Check sheet for the modelled part. Datum: model origin and axes. Units: mm. Give positions to 0.01 mm unless a question says otherwise; leave off trailing zeros. Loops run counter-clockwise (first coordinate to the right, second up) from the corner with the lowest first, then second, coordinate; pieces in that order, holes last. Notation, with made-up numbers: (40.25, 49.25) - (48.25, 49.25) arc R27 cw to (48.25, 85.25) - close; hole circle Ø1 at (43, -3.5). An arc over 180 degrees is marked (long way). Answer in a Markdown table with one row per item. Add a question column.
(1) Sectioned sample at B-B on x = -10.5. Enter the section's corners in (y, z).
(2) Thickness scan on L1, parallel to Y at x = 2, z = -46.5; L2, parallel to X at y = 28, z = -70.5; L3, parallel to Z at x = 0, y = 30. Record the ranges inside material, lowest first.
(3) Sectioned sample at D-D on x = 3. Enter the section's corners in (y, z).
(4) Go/stop test with flat-tipped pins: P1, Ø1.7, axis at x = 22.5, z = 32, coming from the +Y side; P2, Ø2, axis at x = -26.48, z = -26.81, coming from the -Y side. Record where each tip stops, or that it passes through.
(5) Sectioned sample at C-C on y = 15.5. Enter the section's corners in (x, z).
(6) Sectioned sample at A-A on z = -37. Enter the section's corners in (x, y), then the cut area to 3 significant figures.
Autodesk Inventor part; units mm, degrees
ref_plane "YZ Plane" through (0, 0, 0) normal (1, 0, 0) x (0, 1, 0)
ref_plane "XZ Plane" through (0, 0, 0) normal (0, 1, 0) x (-1, 0, 0)
ref_plane "XY Plane" through (0, 0, 0) normal (0, 0, 1) x (1, 0, 0)
sketch "Esquisse1" plane through (0, 0, 0) normal (0, 1, 0) x (-1, 0, 0)
  line L0 (29.9796, 34.6939) -> (-26.0204, 34.6939)
  line L1 (-26.0204, 34.6939) -> (-26.0204, -50.3061)
  line L2 (29.9796, -50.3061) -> (29.9796, 34.6939)
  circle A0 centre (26.4796, 31.1939) radius 1.375
  circle A1 centre (-22.5204, 31.1939) radius 1.375
  circle A2 centre (26.4796, -26.8061) radius 1.375
  circle A3 centre (-22.5204, -26.8061) radius 1.375
  circle A4 centre (26.4796, 31.1939) radius 2.875
  circle A5 centre (-22.5204, 31.1939) radius 2.875
  circle A6 centre (-22.5204, -26.8061) radius 2.875
  circle A7 centre (26.4796, -26.8061) radius 2.875
  line L3 (-26.0204, -50.3061) -> (-26.0204, -90.3061)
  line L4 (-26.0204, -90.3061) -> (29.9796, -90.3061)
  line L5 (29.9796, -90.3061) -> (29.9796, -50.3061)
  line L6 (31.9796, 36.6939) -> (-28.0204, 36.6939)
  line L7 (-28.0204, 36.6939) -> (-28.0204, -92.3061)
  line L8 (-28.0204, -92.3061) -> (31.9796, -92.3061)
  line L9 (31.9796, -92.3061) -> (31.9796, 36.6939)
  point P0 (0, 0)
  dimension "d3" = 2.75
  dimension "d4" = 3.5
  dimension "d5" = 2.75
  dimension "d6" = 3.5
  dimension "d7" = 3.5
  dimension "d8" = 49
  dimension "d9" = 2.75
  dimension "d10" = 58
  dimension "d11" = 3.5
  dimension "d12" = 2.75
  dimension "d13" = 3.5
  dimension "d14" = 58
  dimension "d15" = 5.75
  dimension "d16" = 5.75
  dimension "d17" = 5.75
  dimension "d18" = 5.75
  dimension "d21" = 2
  dimension "d22" = 2
  dimension "d23" = 2
  dimension "d24" = 2
  dimension "d25" = 125
extrude "Extrusion1" add sketch "Esquisse1" along normal blind 2 contours L2 L5 L4 L3 L1 L0 | L9 L8 L7 L6
sketch "Esquisse2" plane through (0, 0, 0) normal (0, -1, 0) x (1, 0, 0)
  circle A0 centre (22.5204, 31.1939) radius 2.875
  circle A1 centre (22.5204, 31.1939) radius 1.375
  circle A2 centre (-26.4796, 31.1939) radius 1.375
  circle A3 centre (22.5204, -26.8061) radius 1.375
  circle A4 centre (-26.4796, -26.8061) radius 1.375
  circle A5 centre (22.5204, -26.8061) radius 2.875
  circle A6 centre (-26.4796, -26.8061) radius 2.875
  circle A7 centre (-26.4796, 31.1939) radius 2.875
  point P0 (0, 0)
  dimension "d28" = 2.75
  dimension "d29" = 2.75
  dimension "d30" = 2.75
  dimension "d31" = 2.75
  dimension "d33" = 0
  dimension "d34" = 0
  dimension "d35" = 0
  dimension "d36" = 0
  dimension "d37" = 0
extrude "Extrusion2" add sketch "Esquisse2" against normal blind 4
sketch "Esquisse3" plane through (0, 2, 0) normal (0, 1, 0) x (1, 0, 0)
  line L0 (-29.9796, -34.6939) -> (26.0204, -34.6939)
  line L1 (26.0204, -34.6939) -> (26.0204, 90.3061)
  line L2 (26.0204, 90.3061) -> (-29.9796, 90.3061)
  line L3 (-29.9796, 90.3061) -> (-29.9796, -34.6939)
  line L4 (-31.9796, 92.3061) -> (-31.9796, -36.6939)
  line L5 (-31.9796, -36.6939) -> (28.0204, -36.6939)
  line L6 (28.0204, 92.3061) -> (-31.9796, 92.3061)
  line L7 (28.0204, -36.6939) -> (28.0204, 92.3061)
  point P0 (0, 0)
  dimension "d40" = 2
  dimension "d41" = 2
  dimension "d42" = 2
  dimension "d43" = 2
extrude "Extrusion3" add sketch "Esquisse3" along normal blind 18
sketch "Esquisse4" plane through (28.0204, 0, -92.3061) normal (0, 0, -1) x (-1, 0, 0)
  line L0 (22, 20) -> (36, 20)
  line L1 (36, 20) -> (36, 5)
  line L2 (36, 5) -> (22, 5)
  line L3 (22, 5) -> (22, 20)
  line L4 (40, 20) -> (54, 20)
  line L5 (54, 20) -> (54, 5)
  line L6 (54, 5) -> (40, 5)
  line L7 (40, 5) -> (40, 20)
  line L8 (0, 0) -> (60, 0)
  line L9 (0, 0) -> (0, 20)
  point P0 (28.0204, 0)
  dimension "d46" = 5
  dimension "d47" = 5
  dimension "d48" = 14
  dimension "d49" = 14
  dimension "d51" = 22
  dimension "d52" = 40
  dimension "d53" = 15
extrude "Extrusion4" cut sketch "Esquisse4" against normal blind 20
sketch "Esquisse5" plane through (28.0204, 0, 36.6939) normal (1, 0, 0) x (0, 0, -1)
  line L0 (12, 8) -> (20, 8)
  line L1 (20, 8) -> (20, 5)
  line L2 (20, 5) -> (12, 5)
  line L3 (12, 5) -> (12, 8)
  line L4 (0, 0) -> (0, 20)
  line L5 (0, 0) -> (129, 0)
  point P0 (36.6939, 0)
  dimension "d56" = 12
  dimension "d57" = 8
  dimension "d58" = 3
  dimension "d59" = 5
extrude "Extrusion5" cut sketch "Esquisse5" against normal blind 20
sketch "Esquisse6" plane through (28.0204, 0, 36.6939) normal (1, 0, 0) x (0, 0, -1)
  line L0 (53, 21) -> (45, 21)
  line L1 (45, 21) -> (45, 18)
  line L2 (45, 18) -> (53, 18)
  line L3 (53, 18) -> (53, 21)
  line L4 (0, 0) -> (129, 0)
  line L5 (0, 20) -> (129, 20)
  line L6 (0, 0) -> (0, 20)
  point P0 (36.6939, 0)
  dimension "d62" = 18
  dimension "d66" = 3
  dimension "d67" = 8
  dimension "d68" = 45
sketch "Esquisse7" plane through (0, 20, 0) normal (0, 1, 0) x (1, 0, 0)
  line L0 (-31.9796, 92.3061) -> (-31.9796, -36.6939)
  line L1 (28.0204, 92.3061) -> (6.0204, 92.3061)
  line L2 (-31.9796, -36.6939) -> (28.0204, -36.6939)
  line L3 (28.0204, -36.6939) -> (28.0204, 92.3061)
  line L4 (28.0204, 92.3061) -> (-31.9796, 92.3061)
  line L5 (-31.9796, 92.3061) -> (-31.9796, -36.6939)
  line L6 (26.0204, 90.3061) -> (-29.9796, 90.3061)
  line L7 (26.0204, 90.3061) -> (26.0204, -34.6939)
  line L8 (-29.9796, 90.3061) -> (26.0204, 90.3061)
  line L9 (26.0204, 90.3061) -> (26.0204, -34.6939)
  line L10 (26.0204, -34.6939) -> (-29.9796, -34.6939)
  line L11 (-29.9796, -34.6939) -> (-29.9796, 90.3061)
  point P0 (0, 0)
extrude "Extrusion6" add sketch "Esquisse7" along normal blind 14
extrude "Extrusion7" cut sketch "Esquisse6" against normal blind 14
sketch "Esquisse8" plane through (0, 34, 0) normal (0, 1, 0) x (1, 0, 0)
  line L0 (-31.9796, 92.3061) -> (-31.9796, -36.6939)
  line L1 (28.0204, -36.6939) -> (28.0204, 92.3061)
  line L2 (-31.9796, -36.6939) -> (28.0204, -36.6939)
  line L3 (28.0204, -36.6939) -> (28.0204, 92.3061)
  line L4 (28.0204, 92.3061) -> (-31.9796, 92.3061)
  line L5 (-31.9796, 92.3061) -> (-31.9796, -36.6939)
  point P0 (0, 0)
extrude "Extrusion8" add sketch "Esquisse8" along normal blind 2
sketch "Esquisse9" plane through (0, 36, 0) normal (0, 1, 0) x (1, 0, 0)
  circle A0 centre (10.0204, -29.6939) radius 5
  line L0 (28.0204, -36.6939) -> (28.0204, 92.3061)
  line L1 (-31.9796, -36.6939) -> (28.0204, -36.6939)
  point P0 (0, 0)
  dimension "d75" = 10
  dimension "d76" = 18
  dimension "d77" = 7
extrude "Extrusion9" cut sketch "Esquisse9" against normal blind 3
sketch "Esquisse10" plane through (0, 36, 0) normal (0, 1, 0) x (1, 0, 0)
  circle A0 centre (23.0204, -30.6939) radius 2.5
  circle A1 centre (10.0204, -29.6939) radius 5
  line L0 (-31.9796, -36.6939) -> (28.0204, -36.6939)
  point P0 (0, 0)
  dimension "d80" = 13
  dimension "d81" = 5
  dimension "d82" = 6
extrude "Extrusion10" cut sketch "Esquisse10" against normal blind 3 contours A0
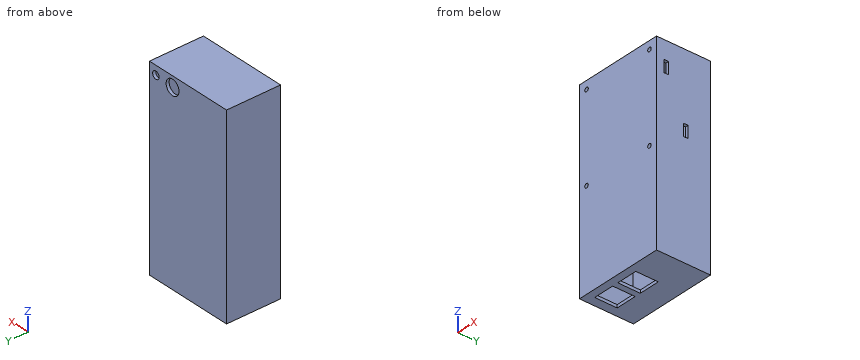
Reply:
| question | item | result |
|---|---|---|
| 1 | outline | (0, -92.31) - (36, -92.31) - (36, 36.69) - (0, 36.69) - close; hole (2, -90.31) - (34, -90.31) - (34, 34.69) - (2, 34.69) - close |
| 2 | L1 | 0 to 2, 34 to 36 |
| 2 | L2 | -31.98 to -29.98, 26.02 to 28.02 |
| 2 | L3 | -92.31 to -90.31, 34.69 to 36.69 |
| 3 | outline | (0, -92.31) - (5, -92.31) - (5, -90.31) - (2, -90.31) - (2, 34.69) - (34, 34.69) - (34, -90.31) - (20, -90.31) - (20, -92.31) - (36, -92.31) - (36, 36.69) - (0, 36.69) - close |
| 4 | P1 | y = 4 |
| 4 | P2 | y = 34 |
| 5 | outline | (-31.98, -92.31) - (-25.98, -92.31) - (-25.98, -90.31) - (-29.98, -90.31) - (-29.98, 34.69) - (26.02, 34.69) - (26.02, -90.31) - (6.02, -90.31) - (6.02, -92.31) - (28.02, -92.31) - (28.02, 36.69) - (-31.98, 36.69) - close; (-11.98, -92.31) - (-7.98, -92.31) - (-7.98, -90.31) - (-11.98, -90.31) - close |
| 6 | outline | (-31.98, 0) - (28.02, 0) - (28.02, 36) - (-31.98, 36) - close; hole (-29.98, 2) - (26.02, 2) - (26.02, 34) - (-29.98, 34) - close |
| 6 | area | 368 mm^2 |
